The model under review builds one solid part; all positions refer to its coordinate system, in mm. Face numbers are marked on the shaded views. A direction names the side the tool comes from. Give positions to 0.01 mm unless a question says otherwise; leave off trailing zeros. Order: outer loops, then holes, each group sorted by start corner. A loop starts at its lowest first (then second) coordinate and runs counter-clockwise, first axis right, second up. Notation, with made-up numbers: (13, 45.25) - (28, 45.25) arc R12 cw to (28, 63.25) - close; hole circle Ø5 at (10, 5). An arc over 180 degrees is marked (long way). Use CSV: the item, a comma, the result in double quotes. Start each with the question number.
1. Draft analysis for pull direction X (two halves, no side actions). For the marked faces 4, 5 and 6, state which applies: released by +X, released by -X, zero draft, split by the parting line, or undercut.
2. Take a section at A-A, the plane x = 141. State the section outline as (y, z) points.
3. Take a section at D-D, the plane x = 63. State the section outline as (y, z) points, then the cut area to 3 significant figures.
4. To check wall thickness, follow line 1 (Y direction, x = 144, z = 12.5); line 2 (X direction, y = 10, z = 40.5); line 3 (Z direction, x = 114, y = 54). State the ranges of each line that lie inside material, in increasing order. Write a range as [from, to].
5. Machinability: for the marked faces 1, 2 and 3, which of the approach directions +Z, -Z, +X, -X, +Y, -Y give a long, thin tool a straight path to every point of the face, cutting with its end or side? Answer none if there is none.
6. Take a section at B-B, the plane y = 32. State the section outline as (x, z) points, then the cut area to 3 significant figures.
7. Take a section at C-C, the plane z = 40.5. State the section outline as (x, y) points, then the cut area to 3 significant figures.
8. For pin 1 (1.5 mm diameter, centred on x = 59.5, z = 40, fed in from -Y); pin 2 (6 mm diameter, centred on x = 87.5, y = 9.5, fed in from +Z); pin 3 (8 mm diameter, centred on y = 42, z = 47.5, fed in from +X); pin 4 (17.5 mm diameter, centred on x = 0, y = 32, fed in from -Z), all flat-tipped, find the tip position at first contact; note any pin that passes through.
Autodesk Fusion 360 part; units mm, degrees
sketch "Sketch1" plane through (0, 0, 0) normal (0, 0, 1) x (1, 0, 0)
  line L0 (0, 0) -> (144, 0)
  line L1 (144, 64) -> (0, 64)
  circle A0 centre (144, 32) radius 11
  circle A1 centre (0, 32) radius 11
  arc A2 (0, 64) -> (0, 0) centre (0, 32) ccw
  arc A3 (144, 0) -> (144, 64) centre (144, 32) ccw
extrude "Extrude1" add sketch "Sketch1" along normal blind 19
sketch "Sketch2" plane through (0, 0, 19) normal (0, 0, 1) x (-1, 0, 0)
  circle A0 centre (-144, -32) radius 11
  circle A1 centre (0, -32) radius 11
  arc A2 (-144, 0) -> (-144, -64) centre (-144, -32) ccw
  line L0 (-144, -64) -> (0, -64)
  arc A3 (0, -64) -> (0, 0) centre (0, -32) ccw
  line L1 (0, 0) -> (-144, 0)
  line L2 (-72, -64) -> (-104, -64)
  line L3 (-104, -64) -> (-104, 0)
  line L4 (-104, 0) -> (-91, 0)
  line L5 (-91, 0) -> (-91, -51)
  line L6 (-91, -51) -> (-72, -51)
  line L7 (-40, 0) -> (-53, 0)
  line L8 (-53, 0) -> (-53, -51)
  line L9 (-53, -51) -> (-72, -51)
  line L10 (-72, -64) -> (-40, -64)
  line L11 (-40, -64) -> (-40, 0)
  dimension "d7" = 32
  dimension "d8" = 13
  dimension "d9" = 51
extrude "Extrude2" add sketch "Sketch2" along normal blind 45 contours L0 L1 L2 L3 L4 L5 L6 L7 L8 L9 L10 L11
sketch "Sketch3" plane through (53, 0, 0) normal (1, 0, 0) x (0, 1, 0)
  line L0 (0, 19) -> (51, 19)
  line L1 (51, 19) -> (51, 64)
  line L2 (51, 64) -> (0, 64)
  line L3 (0, 64) -> (0, 19)
  line L4 (0, 19) -> (51, 64)
  line L5 (51, 64) -> (51, 19)
  line L6 (0, 19) -> (51, 19)
extrude "Extrude3" add sketch "Sketch3" along normal blind 50 contours L0 L1 L4 L5 L6
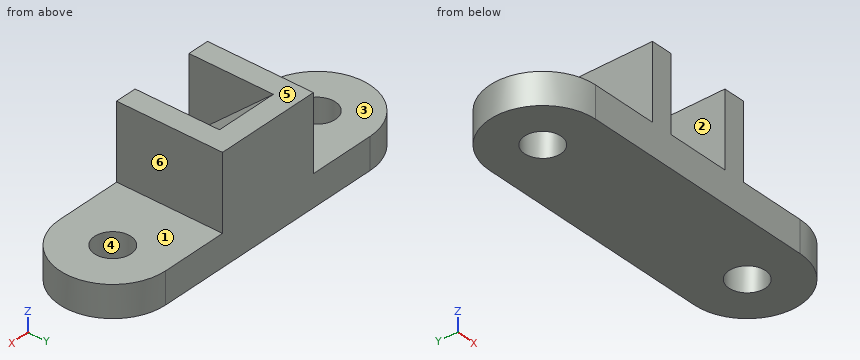
Determined:
1,face 4,"undercut"
1,face 5,"zero draft"
1,face 6,"released by +X"
2,outline,"(0, 0) - (21.42, 0) - (21.42, 19) - (0, 19) - close; (42.58, 0) - (64, 0) - (64, 19) - (42.58, 19) - close"
3,outline,"(0, 0) - (64, 0) - (64, 64) - (51, 64) - (0, 19) - close"
3,area,"2,950 mm²"
4,line 1,"y = [0, 21], [43, 64]"
4,line 2,"x = [40, 53], [91, 104]"
4,line 3,"z = [0, 19]"
5,face 1,"+Z, +X, +Y, -Y"
5,face 2,"+Z, -Y"
5,face 3,"+Z, -X, +Y, -Y"
6,outline,"(-32, 0) - (-11, 0) - (-11, 19) - (-32, 19) - close; (11, 0) - (133, 0) - (133, 19) - (104, 19) - (104, 64) - (91, 64) - (91, 47.24) - (53, 47.24) - (53, 64) - (40, 64) - (40, 19) - (11, 19) - close; (155, 0) - (176, 0) - (176, 19) - (155, 19) - close"
6,area,"5,360 mm²"
7,outline,"(40, 0) - (53, 0) - (53, 24.37) - (91, 24.37) - (91, 0) - (104, 0) - (104, 64) - (40, 64) - close"
7,area,"3,170 mm²"
8,pin 1,"stops at y = 22.95"
8,pin 2,"stops at z = 30.03"
8,pin 3,"stops at x = 104"
8,pin 4,"passes through"
